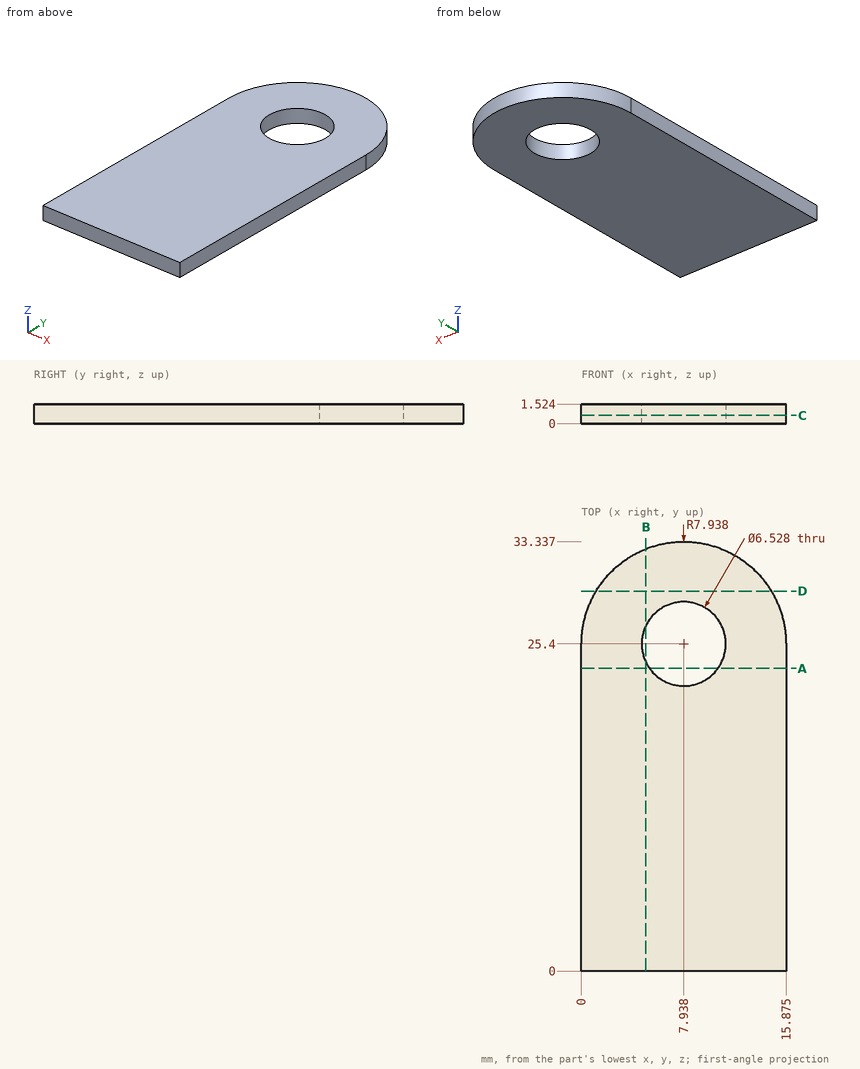
Job drawing, mm, ordinate dimensions from the low corner. One solid piece. Give positions to 0.01 mm unless a question says otherwise; leave off trailing zeros. Write each loop counter-clockwise with the first axis right and the second up, starting at its lowest first coordinate (ties: lowest second). Pieces come first, ordered by that corner, then holes. Notation, with made-up numbers: M -18,-7 L 3,-7 A17 cw 3,23 Z; hole C -11.75,41 d8. An arc over 180 degrees is marked long. One line per item, written item: value. Start each with the question number.
Q1. Saw through at B-B, the plane x = 5. Write the cut outline in (y, z) (1 decimal).
Q2. Saw through at A-A, the plane y = 23.5. Write the cut outline in (x, z) (1 decimal).
Q3. Saw through at D-D, the plane y = 29.5. Write the cut outline in (x, z) (1 decimal), plus the area to 3 significant figures.
Q4. Probe probe 1 along X at (y, z) = (25.4, 0.95) (1 decimal); probe 2 along X at (y, z) = (26.5, 0.85) (1 decimal); probe 3 along Y at (x, z) = (9, 0.8) (1 decimal). List the from-to ranges inside material, lowest first. Write a range as [from, to].
Q5. Saw through at C-C, the plane z = 0.65. Write the cut outline in (x, y) (1 decimal).
Output values:
1. outline: M 0,0 L 24,0 L 24,1.5 L 0,1.5 Z; M 26.8,0 L 32.8,0 L 32.8,1.5 L 26.8,1.5 Z
2. outline: M 0,0 L 5.3,0 L 5.3,1.5 L 0,1.5 Z; M 10.6,0 L 15.9,0 L 15.9,1.5 L 10.6,1.5 Z
3. outline: M 1.1,0 L 14.7,0 L 14.7,1.5 L 1.1,1.5 Z
3. area: 20.7 mm²
4. probe 1: x = [0, 4.7], [11.2, 15.9]
4. probe 2: x = [0.1, 4.9], [11, 15.8]
4. probe 3: y = [0, 22.3], [28.5, 33.3]
5. outline: M 0,0 L 15.9,0 L 15.9,25.4 A7.9 ccw 0,25.4 Z; hole C 7.9,25.4 d6.5
